```python
from build123d import *

# Parameters (mm, degrees)
SKETCH_W        = 195
SKETCH_H        = 120
PAD_DEPTH       = 3
SKETCH001_R     = 1.6
POCKET_DEPTH    = 5
SKETCH002_R     = 2.5
SKETCH002_R_2   = 2.1
POCKET001_DEPTH = 5


with BuildPart() as part:
    # Sketch → Pad (new body)
    with BuildSketch(Plane.XY):
        Rectangle(SKETCH_W, SKETCH_H)
    extrude(amount=PAD_DEPTH)

    # Sketch001 → Pocket (cut)
    with BuildSketch(Plane.XY.offset(3)):
        with Locations((-90.75, 57.9)):
            Circle(SKETCH001_R)
        with Locations((90.75, 57.9)):
            Circle(SKETCH001_R)
        with Locations((-90.75, -57.9)):
            Circle(SKETCH001_R)
        with Locations((90.75, -57.9)):
            Circle(SKETCH001_R)
    extrude(amount=-POCKET_DEPTH, mode=Mode.SUBTRACT)

    # Sketch002 → Pocket001 (cut)
    with BuildSketch(Plane.XY.offset(3)):
        with Locations((-57.2, -40)):
            Circle(SKETCH002_R)
        with Locations((-28.6, -40)):
            Circle(SKETCH002_R)
        with Locations((0, -40)):
            Circle(SKETCH002_R)
        with Locations((28.6, -40)):
            Circle(SKETCH002_R)
        with Locations((57.2, -40)):
            Circle(SKETCH002_R)
        with Locations((-80.965, 42.9)):
            Circle(SKETCH002_R_2)
        with Locations((-80.965, 35)):
            Circle(SKETCH002_R_2)
        with Locations((80.965, 42.9)):
            Circle(SKETCH002_R_2)
        with Locations((80.965, 35)):
            Circle(SKETCH002_R_2)
        with Locations((-85.8, -40)):
            Circle(SKETCH002_R)
        with Locations((85.8, -40)):
            Circle(SKETCH002_R)
    extrude(amount=-POCKET001_DEPTH, mode=Mode.SUBTRACT)


solid = part.part
```
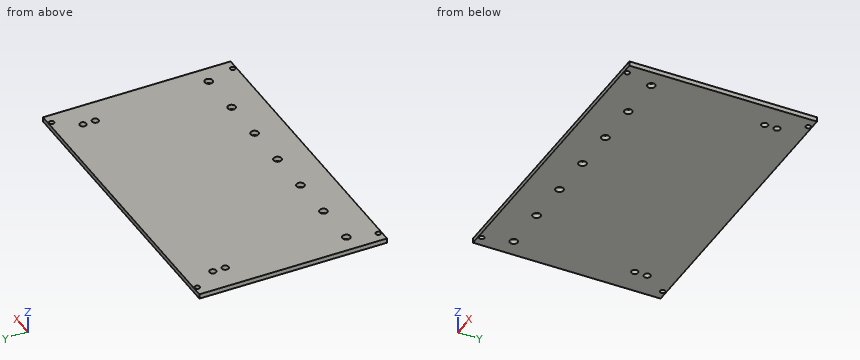
CAD build for the part. Positions are in the model's coordinates, mm. Give positions to 0.01 mm unless a question says otherwise; leave off trailing zeros. Order: outer loops, then holes, each group sorted by start corner. A loop starts at its lowest first (then second) coordinate and runs counter-clockwise, first axis right, second up.
(1) Saw through at C-C, the plane y = 35. Give the cut face in (x, z) (3 decimals).
(2) Saw through at B-B, the plane x = -85.8. Give the cut face in (y, z).
(3) Drill centre lines: L1, parallel to Y at x = -90.75, z = 0.75; L2, parallel to Y at x = 57.2, z = 1.05; L3, parallel to Y at x = -84.5, z = 1.4. Where is each one in solid material? Low to high.
(4) Saw through at A-A, the plane y = -40. State how many separate pieces and enclosed holes the cut face has, then the cut area to 3 significant figures.
Results found:
1. outline: (-97.5, 0) - (-83.065, 0) - (-83.065, 3) - (-97.5, 3) - close; (-78.865, 0) - (78.865, 0) - (78.865, 3) - (-78.865, 3) - close; (83.065, 0) - (97.5, 0) - (97.5, 3) - (83.065, 3) - close
2. outline: (-60, 0) - (-42.5, 0) - (-42.5, 3) - (-60, 3) - close; (-37.5, 0) - (60, 0) - (60, 3) - (-37.5, 3) - close
3. L1: y = -60 to -59.5, -56.3 to 56.3, 59.5 to 60
3. L2: y = -60 to -42.5, -37.5 to 60
3. L3: y = -60 to -42.14, -37.86 to 60
4. separate pieces: 8
4. enclosed holes: 0
4. area: 480 mm2
